CAD build for the part. Positions are in the model's coordinates, mm. A direction names the side the tool comes from. Give positions to 0.01 mm unless a question says otherwise; leave off trailing zeros. Write each loop counter-clockwise with the first axis right and the second up, starting at its lowest first coordinate (ties: lowest second). Pieces come first, ordered by that corner, then holes. Notation, with made-up numbers: (34, 5.5) - (38, 5.5) arc R21 ccw to (38, 18.5) - close; hole circle Ø11 at (-40, -22.75). An arc over 180 degrees is marked (long way). Put each result on its own line as item: value. Start each with the question number.
1. Cut at B-B on y = 40.5. List the corners of the cut face in (x, z).
2. Cut at A-A on y = 52. List the corners of the cut face in (x, z).
3. Drop flat-ended pins along their axis: pin 1 (1.5 mm diameter, centred on x = 5.5, z = 4.5, fed in from +Y); pin 2 (12 mm diameter, centred on x = 52.5, y = 20.5, fed in from +Z); pin 3 (1.5 mm diameter, centred on x = -15, z = 12.5, fed in from -Y); pin 4 (3 mm diameter, centred on y = 52, z = 14, fed in from -X). Give the stop position or say it passes through.
4. Mould opens along Z. For faces 5 (the flat face through (-16, 3, 11)), 6 (the flat face through (-2, 3, 16)), 7 (the flat face through (-8, 3, 4)) say: +Z half, -Z half, draft (parallel to the pull), parting line (faces both ways), or undercut.
5. Wall check: line 1 (Y direction, x = 8.15, z = 15.5); line 2 (X direction, y = 51, z = 3.25); line 3 (Y direction, x = -26.35, z = 14). Give the ranges that are in metal, low to high.
6. Cut at D-D on z = 13.5. Give the number of separate pieces and of enclosed holes in the cut face, and give its area (3 significant figures).
7. Tool access for faces 1 (the flat face through (33, 24.75, 9)), 2 (the flat face through (58, 10, 8)), 3 (the flat face through (0, 27, 9)), 4 (the flat face through (-2, 52, 2)): list every direction of +Z, -Z, +X, -X, +Y, -Y with a clear straight run to the whole face (end or side of a thin tool).
8. Cut at C-C on x = 8.15. List the corners of the cut face in (y, z).
from build123d import *

# Parameters (mm, degrees)
SKETCH2_W               = 66
SKETCH2_H               = 55
SKETCH2_W_2             = 42
SKETCH2_H_2             = 20.5
SKETCH2_W_3             = 42.5
BOSS_EXTRUDE1_DEPTH     = 18
SKETCH3_R               = 2.5
CUT_EXTRUDE1_DEPTH      = 10
SKETCH5_W               = 2
SKETCH5_H               = 6
BOSS_EXTRUDE2_DEPTH     = 26.8
BOSS_EXTRUDE3_REACH     = 89.39
SKETCH6_W               = 3
SKETCH6_H               = 6
SKETCH6_W_2             = 2
SKETCH7_R               = 1.6
CUT_EXTRUDE2_DEPTH      = 10
CUT_EXTRUDE3_REACH      = 89.778
SKETCH8_W               = 42
SKETCH8_H               = 4.25
SKETCH8_W_2             = 42.5
SKETCH9_W               = 3
SKETCH9_H               = 6
BOSS_EXTRUDE5_DEPTH     = 14
CUT_EXTRUDE4_DEPTH      = 21
CUT_EXTRUDE4_DEPTH_BACK = 10
SKETCH10_W              = 15.8
SKETCH10_H              = 6.002189295
SKETCH11_W              = 4
SKETCH11_H              = 6
BOSS_EXTRUDE6_DEPTH     = 15.8
SKETCH12_W              = 3
SKETCH12_H              = 6
BOSS_EXTRUDE7_DEPTH     = 14
CUT_EXTRUDE5_DEPTH      = 18
CUT_EXTRUDE5_DEPTH_BACK = 10
SKETCH13_W              = 16.8
SKETCH13_H              = 6
SKETCH14_W              = 4
SKETCH14_H              = 6
BOSS_EXTRUDE8_DEPTH     = 16.8


with BuildPart() as part:
    # Sketch2 → Boss-Extrude1 (new body)
    with BuildSketch(Plane.XY):
        with Locations((33, 27.5)):
            Rectangle(SKETCH2_W, SKETCH2_H)
        with Locations((33, 40.5)):
            Rectangle(SKETCH2_W_2, SKETCH2_H_2, mode=Mode.SUBTRACT)
        with Locations((33.25, 14.5)):
            Rectangle(SKETCH2_W_3, SKETCH2_H_2, mode=Mode.SUBTRACT)
    extrude(amount=BOSS_EXTRUDE1_DEPTH)

    # Sketch3 → Cut-Extrude1 (cut)
    with BuildSketch(Plane.XY.offset(18)):
        with Locations((8.15, 45.75)):
            Circle(SKETCH3_R)
        with Locations((8.15, 35.75)):
            Circle(SKETCH3_R)
        with Locations(Location((57.85, 35.75, 0), (0, 0, 180))):
            Circle(SKETCH3_R)
        with Locations(Location((57.85, 45.75, 0), (0, 0, 180))):
            Circle(SKETCH3_R)
        with Locations(Location((8.15, 19.75, 0), (0, 0, 180))):
            Circle(SKETCH3_R)
        with Locations(Location((8.15, 9.75, 0), (0, 0, 180))):
            Circle(SKETCH3_R)
        with Locations((57.85, 9.75)):
            Circle(SKETCH3_R)
        with Locations((57.85, 19.75)):
            Circle(SKETCH3_R)
    extrude(amount=-CUT_EXTRUDE1_DEPTH, mode=Mode.SUBTRACT)

    # Sketch5 → Boss-Extrude2 (add)
    with BuildSketch(Plane.ZY):
        with Locations((1, 52)):
            Rectangle(SKETCH5_W, SKETCH5_H)
        with Locations((17, 52)):
            Rectangle(SKETCH5_W, SKETCH5_H)
        with Locations((1, 3)):
            Rectangle(SKETCH5_W, SKETCH5_H)
        with Locations((17, 3)):
            Rectangle(SKETCH5_W, SKETCH5_H)
    extrude(amount=BOSS_EXTRUDE2_DEPTH)

    # Sketch6 → Boss-Extrude3 (add, up to next)
    with BuildSketch(Plane.XY.offset(2), mode=Mode.PRIVATE) as boss_extrude3_sk1:
        with Locations((-25.3, 52)):
            Rectangle(SKETCH6_W, SKETCH6_H)
    boss_extrude3_tool1 = extrude(boss_extrude3_sk1.sketch, amount=BOSS_EXTRUDE3_REACH, mode=Mode.PRIVATE) - part.part
    # Sketch6 → Boss-Extrude3 (add, up to next)
    with BuildSketch(Plane.XY.offset(2), mode=Mode.PRIVATE) as boss_extrude3_sk2:
        with Locations((-25.8, 3)):
            Rectangle(SKETCH6_W_2, SKETCH6_H)
    boss_extrude3_tool2 = extrude(boss_extrude3_sk2.sketch, amount=BOSS_EXTRUDE3_REACH, mode=Mode.PRIVATE) - part.part
    add(boss_extrude3_tool1.solids().sort_by_distance((-25.3, 52, 2))[0])
    add(boss_extrude3_tool2.solids().sort_by_distance((-25.8, 3, 2))[0])

    # Sketch7 → Cut-Extrude2 (cut)
    with BuildSketch(Plane.ZY.offset(26.8)):
        with Locations((4, 52)):
            Circle(SKETCH7_R)
        with Locations((14, 52)):
            Circle(SKETCH7_R)
        with Locations((4, 3)):
            Circle(SKETCH7_R)
        with Locations((14, 3)):
            Circle(SKETCH7_R)
    extrude(amount=-CUT_EXTRUDE2_DEPTH, mode=Mode.SUBTRACT)

    # Sketch8 → Cut-Extrude3 (cut, up to next)
    with BuildSketch(Plane.XY.offset(18), mode=Mode.PRIVATE) as cut_extrude3_sk1:
        with Locations((33, 52.875)):
            Rectangle(SKETCH8_W, SKETCH8_H)
    cut_extrude3_tool1 = extrude(cut_extrude3_sk1.sketch, amount=-CUT_EXTRUDE3_REACH, mode=Mode.PRIVATE) & part.part
    # Sketch8 → Cut-Extrude3 (cut, up to next)
    with BuildSketch(Plane.XY.offset(18), mode=Mode.PRIVATE) as cut_extrude3_sk2:
        with Locations((33.25, 2.125)):
            Rectangle(SKETCH8_W_2, SKETCH8_H)
    cut_extrude3_tool2 = extrude(cut_extrude3_sk2.sketch, amount=-CUT_EXTRUDE3_REACH, mode=Mode.PRIVATE) & part.part
    add(cut_extrude3_tool1.solids().sort_by_distance((33, 52.875, 18))[0], mode=Mode.SUBTRACT)
    add(cut_extrude3_tool2.solids().sort_by_distance((33.25, 2.125, 18))[0], mode=Mode.SUBTRACT)

    # Sketch9 → Boss-Extrude5 (add)
    with BuildSketch(Plane.XY.offset(2)):
        with Locations((-6.5, 52.002189295)):
            Rectangle(SKETCH9_W, SKETCH9_H)
    extrude(amount=BOSS_EXTRUDE5_DEPTH)

    # Sketch10 → Cut-Extrude4 (cut, two sides: drawn at the far end of the back side and taken through both)
    with BuildSketch(Plane(origin=(0, 0, 16), x_dir=(-1, 0, 0), z_dir=(0, 0, -1)).offset(-CUT_EXTRUDE4_DEPTH_BACK)):
        with Locations((15.9, 52.001094647)):
            Rectangle(SKETCH10_W, SKETCH10_H)
    extrude(amount=CUT_EXTRUDE4_DEPTH + CUT_EXTRUDE4_DEPTH_BACK, mode=Mode.SUBTRACT)


with BuildPart() as cut_extrude4_piece_1:
    # of the separate pieces the step leaves, piece 1, a body of its own (cut_extrude4_pieces)
    add(part.part.solids().sort_by_distance((12, 55, 0))[0])



with BuildPart() as cut_extrude4_piece_2:
    # of the separate pieces the step leaves, piece 2, a body of its own (cut_extrude4_pieces)
    add(part.part.solids().sort_by_distance((-23.8, 55, 0))[0])


with BuildPart() as cut_extrude4_piece_1_1:
    add(cut_extrude4_piece_1.part)

    add(cut_extrude4_piece_2.part)  # Boss-Extrude6 merges Cut-Extrude4 piece 2
    # Sketch11 → Boss-Extrude6 (add)
    with BuildSketch(Plane.ZY.offset(8)):
        with Locations((9, 52)):
            Rectangle(SKETCH11_W, SKETCH11_H)
    extrude(amount=BOSS_EXTRUDE6_DEPTH)

    # Sketch12 → Boss-Extrude7 (add)
    with BuildSketch(Plane.XY.offset(2)):
        with Locations((-6.5, 3)):
            Rectangle(SKETCH12_W, SKETCH12_H)
    extrude(amount=BOSS_EXTRUDE7_DEPTH)

    # Sketch13 → Cut-Extrude5 (cut, two sides: drawn at the far end of the back side and taken through both)
    with BuildSketch(Plane(origin=(0, 0, 16), x_dir=(-1, 0, 0), z_dir=(0, 0, -1)).offset(-CUT_EXTRUDE5_DEPTH_BACK)):
        with Locations((16.4, 3)):
            Rectangle(SKETCH13_W, SKETCH13_H)
    extrude(amount=CUT_EXTRUDE5_DEPTH + CUT_EXTRUDE5_DEPTH_BACK, mode=Mode.SUBTRACT)


with BuildPart() as cut_extrude5_piece_1:
    # of the separate pieces the step leaves, piece 1, a body of its own (cut_extrude5_pieces)
    add(cut_extrude4_piece_1_1.part.solids().sort_by_distance((-23.8, 55, 0))[0])



with BuildPart() as cut_extrude5_piece_2:
    # of the separate pieces the step leaves, piece 2, a body of its own (cut_extrude5_pieces)
    add(cut_extrude4_piece_1_1.part.solids().sort_by_distance((-24.8, 0, 18))[0])


with BuildPart() as cut_extrude5_piece_1_1:
    add(cut_extrude5_piece_1.part)

    add(cut_extrude5_piece_2.part)  # Boss-Extrude8 merges Cut-Extrude5 piece 2
    # Sketch14 → Boss-Extrude8 (add)
    with BuildSketch(Plane.ZY.offset(8)):
        with Locations((9, 3)):
            Rectangle(SKETCH14_W, SKETCH14_H)
    extrude(amount=BOSS_EXTRUDE8_DEPTH)


solid = cut_extrude5_piece_1_1.part
Report:
1. outline: (0, 0) - (12, 0) - (12, 18) - (0, 18) - close; (54, 0) - (66, 0) - (66, 18) - (54, 18) - close
2. outline: (-26.8, 0) - (-23.8, 0) - (-23.8, 2.4) - (-26.8, 2.4) - close; (-26.8, 5.6) - (-23.8, 5.6) - (-23.8, 7) - (-8, 7) - (-8, 0) - (12, 0) - (12, 18) - (-8, 18) - (-8, 11) - (-23.8, 11) - (-23.8, 12.4) - (-26.8, 12.4) - close; (-26.8, 15.6) - (-23.8, 15.6) - (-23.8, 18) - (-26.8, 18) - close; (54, 0) - (66, 0) - (66, 18) - (54, 18) - close; hole (-5, 2) - (0, 2) - (0, 16) - (-5, 16) - close
3. pin 1: stops at y = 55
3. pin 2: stops at z = 18
3. pin 3: passes through
3. pin 4: stops at x = -8
4. face 5: +Z half
4. face 6: undercut
4. face 7: draft
5. line 1: y = 0 to 7.25, 12.25 to 17.25, 22.25 to 33.25, 38.25 to 43.25, 48.25 to 55
5. line 2: x = -8 to -5, 0 to 12, 54 to 66
5. line 3: y = 0 to 1.4, 4.6 to 6, 49 to 50.4, 53.6 to 55
6. separate pieces: 7
6. enclosed holes: 8
6. area: 1,430 mm²
7. face 1: +Z, -Z, -Y
7. face 2: +Z
7. face 3: none
7. face 4: +Y, -Y
8. outline: (0, 0) - (55, 0) - (55, 18) - (48.25, 18) - (48.25, 8) - (43.25, 8) - (43.25, 18) - (38.25, 18) - (38.25, 8) - (33.25, 8) - (33.25, 18) - (22.25, 18) - (22.25, 8) - (17.25, 8) - (17.25, 18) - (12.25, 18) - (12.25, 8) - (7.25, 8) - (7.25, 18) - (0, 18) - close
